Part model, mm, in its own coordinate system. A direction names the side the tool comes from. Give positions to 0.01 mm unless a question says otherwise; leave off trailing zeros. Loops run counter-clockwise (first coordinate to the right, second up) from the corner with the lowest first, then second, coordinate; pieces in that order, holes last. Notation, with made-up numbers: (-39, 70) -> (-33, 70) arc R9 cw to (-33, 85) -> close; hole circle Ø3 at (-30.75, 58). An arc over 180 degrees is marked (long way). One line per question, with ' | ' between items.
```python
from build123d import *

# Parameters (mm, degrees)
SKETCH1_W           = 38.1
SKETCH1_H           = 7.62
BOSS_EXTRUDE1_DEPTH = 12.7
SKETCH2_W           = 39.624
SKETCH2_H           = 25.4
BOSS_EXTRUDE2_DEPTH = 12.7
SKETCH3_R           = 2.032
CUT_EXTRUDE1_DEPTH  = 7.62


with BuildPart() as part:
    # Sketch1 → Boss-Extrude1 (new body)
    with BuildSketch(Plane.XY):
        with Locations((-19.05, 3.81)):
            Rectangle(SKETCH1_W, SKETCH1_H)
    extrude(amount=BOSS_EXTRUDE1_DEPTH)

    # Sketch2 → Boss-Extrude2 (add)
    with BuildSketch(Plane.XY.offset(12.7)):
        with Locations((-18.288, 3.81)):
            Rectangle(SKETCH2_W, SKETCH2_H)
    extrude(amount=BOSS_EXTRUDE2_DEPTH)

    # Sketch3 → Cut-Extrude1 (cut)
    with BuildSketch(Plane.XY.offset(25.4)):
        with Locations((-33.909, 13.462)):
            Circle(SKETCH3_R)
        with Locations((-23.495, 13.462)):
            Circle(SKETCH3_R)
        with Locations((-2.667, 13.462)):
            Circle(SKETCH3_R)
        with Locations((-13.081, 2.794)):
            Circle(SKETCH3_R)
        with Locations((-23.495, 2.794)):
            Circle(SKETCH3_R)
        with Locations((-33.909, 2.794)):
            Circle(SKETCH3_R)
        with Locations((-13.081, 13.462)):
            Circle(SKETCH3_R)
        with Locations((-2.667, 2.794)):
            Circle(SKETCH3_R)
    extrude(amount=-CUT_EXTRUDE1_DEPTH, mode=Mode.SUBTRACT)


solid = part.part
```
1) Pin check, flat tips, straight feed: P1, Ø2.5, axis at x = -33.909, y = 13.462, coming from the +Z side; P2, Ø6.5, axis at x = -23.495, y = 13.462, coming from the -Z side; P3, Ø10, axis at x = -18.5, z = 3.5, coming from the +Y side. Stop position of each tip, or through.
Found:
P1: z = 17.78 | P2: z = 12.7 | P3: y = 7.62
2) Saw through at C-C (y = 4). Give the cut face in (x, z).
Found:
outline: (-38.1, 0) -> (0, 0) -> (0, 12.7) -> (1.52, 12.7) -> (1.52, 25.4) -> (-1.03, 25.4) -> (-1.03, 17.78) -> (-4.3, 17.78) -> (-4.3, 25.4) -> (-11.45, 25.4) -> (-11.45, 17.78) -> (-14.72, 17.78) -> (-14.72, 25.4) -> (-21.86, 25.4) -> (-21.86, 17.78) -> (-25.13, 17.78) -> (-25.13, 25.4) -> (-32.27, 25.4) -> (-32.27, 17.78) -> (-35.54, 17.78) -> (-35.54, 25.4) -> (-38.1, 25.4) -> close
3) Drill centre lines: line 1 (Y direction, x = -34, z = 24.25); line 2 (Z direction, x = -13.5, y = -3.25); line 3 (Y direction, x = -24, z = 7.75). Where is each one in solid material? Low to high.
Found:
line 1: -8.89 to 0.76, 4.82 to 11.43, 15.49 to 16.51 | line 2: 12.7 to 25.4 | line 3: 0 to 7.62
4) Saw through at D-D (z = 9.25). Give the cut face in (x, y), and give its area (3 significant figures).
Found:
outline: (-38.1, 0) -> (0, 0) -> (0, 7.62) -> (-38.1, 7.62) -> close | area: 290 mm2
5) Saw through at B-B (x = -17.5). Give the cut face in (y, z).
Found:
outline: (-8.89, 12.7) -> (0, 12.7) -> (0, 0) -> (7.62, 0) -> (7.62, 12.7) -> (16.51, 12.7) -> (16.51, 25.4) -> (-8.89, 25.4) -> close
6) Pull direction Y, two halves, no side cores. Call faces 4 (the cylindrical face through (-1.73, 11.66, 21.64)), 5 (the flat face through (-19, 0, 6)), 6 (the flat face through (-13, 3, 17.78)), 7 (the flat face through (-38.1, 4, 15)): pulls with the +Y half, pulls with the -Y half, needs draft (parallel to the pull), parting line crosses it, or undercut.
Found:
face 4: undercut | face 5: pulls with the -Y half | face 6: undercut | face 7: needs draft
7) Saw through at A-A (z = 21.25). State how many separate pieces and enclosed holes the cut face has, and give its area (3 significant figures).
Found:
separate pieces: 1 | enclosed holes: 8 | area: 903 mm2
8) Tool access for faces 1 (the flat face through (-19, 16.51, 19)), 2 (the flat face through (0, 4, 6)), 3 (the cylindrical face through (-13.52, 11.48, 21.64)): list every direction of +Z, -Z, +X, -X, +Y, -Y with a clear straight run to the whole face (end or side of a thin tool).
Found:
face 1: +Z, -Z, +X, -X, +Y | face 2: -Z, +X, +Y, -Y | face 3: +Z
